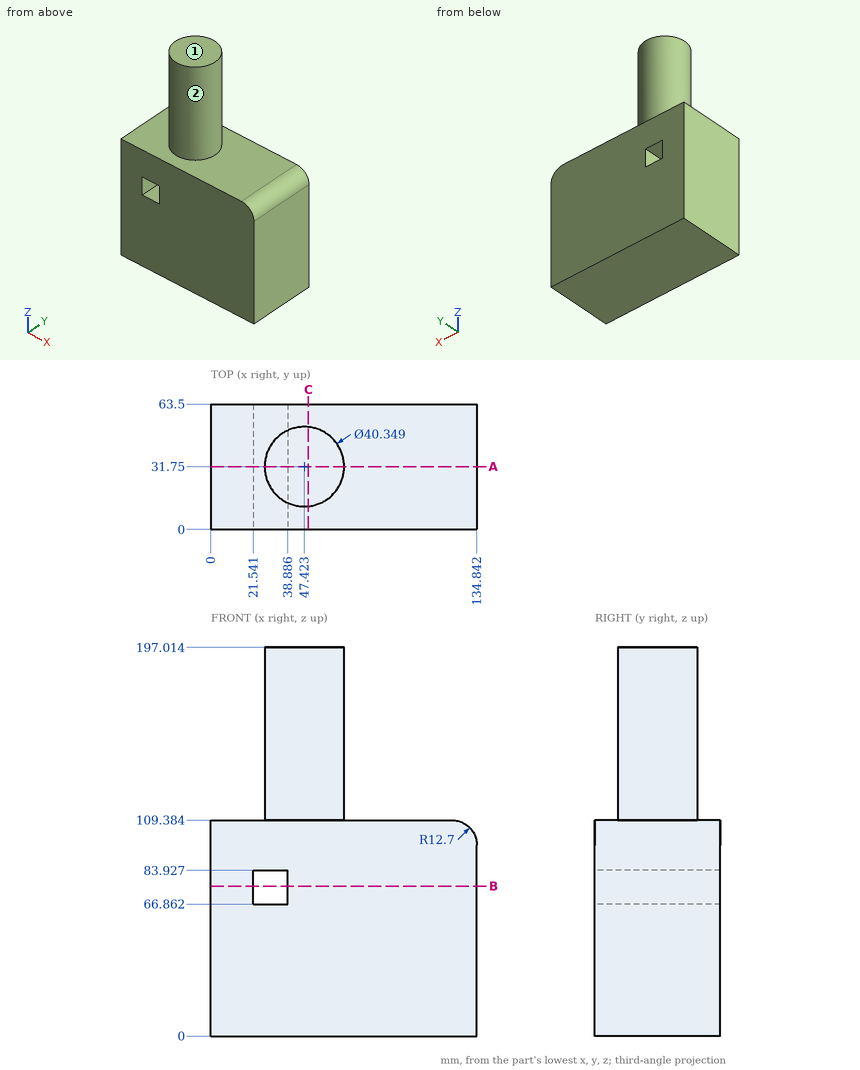
Here's the drawing with two shaded views (mm, measured from the low corner). I have some questions. A direction names the side the tool comes from. Round coordinates to 2 decimals unless told otherwise and drop trailing zeros. Loops run counter-clockwise (first coordinate to the right, second up) from the corner with the lowest first, then second, coordinate; pieces in that order, holes last. Notation, with made-up numbers: M 63,-31 L 84,-31 A24 cw 84,-4 Z; hole C -31,8.25 d2. An arc over 180 degrees is marked long. Answer as a JSON object with one key per item and string values. Group by question number.
Q1. Will these pins go through, and if not, where does the flat tip stop? pin 1 (5 mm diameter, centred on y = 34, z = 47, fed in from -X); pin 2 (4 mm diameter, centred on y = 12, z = 167.5, fed in from -X) (1 decimal); pin 3 (1 mm diameter, centred on y = 25, z = 108, fed in from +X).
Q2. Imagine slicing it at C-C, the plane x = 49.5. Please give me the cut outline in (y, z) (1 decimal), then the cut area to 3 significant figures.
Q3. Imagine slicing it at B-B, the plane z = 76. Please give me the cut outline in (x, y) (1 decimal), then the cut area to 3 significant figures.
Q4. Imagine slicing it at A-A, the plane y = 31.75. Please give me the cut outline in (x, z) (1 decimal), then the cut area to 3 significant figures.
Q5. Please list where these lines run through material, in increasing order: L1, parallel to Z at x = 23.5, y = 58.5 (1 decimal); L2, parallel to X at y = 22.5, z = 83 (1 decimal); L3, parallel to Z at x = 32, y = 38 (1 decimal).
Q6. On a 3-axis mill with a long thin cutter (end or side, diameter ignored), from which of +Z, -Z, +X, -X, +Y, -Y can I reach the whole of each face in a straight line? I mean the marked faces 1 and 2. Say none if no direction works.
Findings:
{
 "1": {"pin 1": "stops at x = 0", "pin 2": "stops at x = 37.8", "pin 3": "stops at x = 128.8"},
 "2": {"outline": "M 0,0 L 63.5,0 L 63.5,109.4 L 51.8,109.4 L 51.8,197 L 11.7,197 L 11.7,109.4 L 0,109.4 Z", "area": "10,500 mm2"},
 "3": {"outline": "M 0,0 L 21.5,0 L 21.5,63.5 L 0,63.5 Z; M 38.9,0 L 134.8,0 L 134.8,63.5 L 38.9,63.5 Z", "area": "7,460 mm2"},
 "4": {"outline": "M 0,0 L 134.8,0 L 134.8,96.7 A12.7 ccw 122.1,109.4 L 67.6,109.4 L 67.6,197 L 27.2,197 L 27.2,109.4 L 0,109.4 Z; hole M 21.5,66.9 L 38.9,66.9 L 38.9,83.9 L 21.5,83.9 Z", "area": "18,000 mm2"},
 "5": {"L1": "z = 0 to 66.9, 83.9 to 109.4", "L2": "x = 0 to 21.5, 38.9 to 134.8", "L3": "z = 0 to 66.9, 83.9 to 197"},
 "6": {"face 1": "+Z, +X, -X, +Y, -Y", "face 2": "+Z"}
}
